The listing builds one solid part. Answer for the finished solid, in the listing's coordinates (mm). Give positions to 0.01 mm unless a question says otherwise; leave off trailing zeros. Order: outer loops, then holes, each group sorted by start corner. A loop starts at its lowest first (then second) coordinate and runs counter-clockwise, first axis right, second up. Notation, with made-up numbers: (-19.75, -27) - (3.25, -27) arc R22 ccw to (3.25, -8) - close; hole circle Ø6 at (-23, 76.5). An arc over 180 degrees is marked (long way). Answer as a JSON object with one key per item and string values. Group by question number.
Q1. A cutting plane is placed at A-A, the plane y = 0.75. Give the vertices of the cut face in (x, z) (3 decimals).
Q2. Consider line 1 (X direction, y = 2.45, z = -209.55) (3 decimals); line 2 (X direction, y = 2.45, z = 10.5); line 3 (X direction, y = 2.1, z = -142). Determine where each line is inside the solid, lowest interval first.
Q3. A cutting plane is placed at C-C, the plane x = -142.5. Give the vertices of the cut face in (y, z).
Q4. A cutting plane is placed at B-B, the plane z = 39. Give the vertices of the cut face in (x, y).
Q5. Given pin 1 (5 mm diameter, centred on x = 181.48, z = 104.78, fed in from -Y), flat-ended and moving along its own axis, determine where the tip first touches the part or whether it passes through.
from build123d import *

# Parameters (mm, degrees)
BOSS_EXTRUDE1_DEPTH = 4.7625
SKETCH2_R           = 3.175
CUT_EXTRUDE1_DEPTH  = 337.044165857


with BuildPart() as part:
    # Sketch1 → Boss-Extrude1 (new body)
    with BuildSketch(Plane(origin=(0, 0, 0), x_dir=(1, 0, 0), z_dir=(0, 1, 0))):
        Polygon((0, 254), (-219.970452561, -127), (219.970452561, -127), align=None)
    extrude(amount=BOSS_EXTRUDE1_DEPTH)

    # Sketch2 → Cut-Extrude1 (cut, through all)
    with BuildSketch(Plane(origin=(0, 4.7625, 0), x_dir=(1, 0, 0), z_dir=(0, 1, 0))):
        with Locations(Location((0, 209.55, 0), (0, 0, 270))):
            Circle(SKETCH2_R)
        with Locations(Location((-181.475623363, -104.775, 0), (0, 0, 270))):
            Circle(SKETCH2_R)
        with Locations(Location((181.475623363, -104.775, 0), (0, 0, 270))):
            Circle(SKETCH2_R)
    extrude(amount=-CUT_EXTRUDE1_DEPTH, mode=Mode.SUBTRACT)


solid = part.part
Reply:
{
 "1": {"outline": "(-219.97, 127) - (0, -254) - (219.97, 127) - close; hole circle Ø6.35 at (-181.476, 104.775); hole circle Ø6.35 at (0, -209.55); hole circle Ø6.35 at (181.476, 104.775)"},
 "2": {"line 1": "x = -25.663 to -3.175, 3.175 to 25.663", "line 2": "x = -152.71 to 152.71", "line 3": "x = -64.66 to 64.66"},
 "3": {"outline": "(0, -7.18) - (4.76, -7.18) - (4.76, 127) - (0, 127) - close"},
 "4": {"outline": "(-169.16, 0) - (169.16, 0) - (169.16, 4.76) - (-169.16, 4.76) - close"},
 "5": {"pin 1": "passes through"}
}
